from build123d import *

# Parameters (mm, degrees)
SKETCH1_W                  = 92
SKETCH1_H                  = 62
BOSS_EXTRUDE1_DEPTH        = 1
F_2_2_2_2_DIAMETER_HOLE2_D = 2.2


with BuildPart() as part:
    # Sketch1 → Boss-Extrude1 (new body)
    with BuildSketch(Plane.XY):
        with Locations((46, -31)):
            Rectangle(SKETCH1_W, SKETCH1_H)
    extrude(amount=-BOSS_EXTRUDE1_DEPTH)

    # Ø2.2 (2.2) Diameter Hole2 (through all)
    with Locations(Plane(origin=(0, 0, -1), x_dir=(-1, 0, 0), z_dir=(0, 0, -1))):
        with Locations((-79, -2), (-57, -2), (-35, -2), (-13, -2), (-13, -60), (-35, -60), (-57, -60), (-79, -60)):
            Hole(F_2_2_2_2_DIAMETER_HOLE2_D / 2)


solid = part.part
Input: part model. Units: mm. Frame: model coordinates. Give positions to 0.01 mm unless a question says otherwise; leave off trailing zeros. Order: outer loops, then holes, each group sorted by start corner. A loop starts at its lowest first (then second) coordinate and runs counter-clockwise, first axis right, second up. Notation, with made-up numbers: (28, -23.5) - (83, -23.5) arc R12 ccw to (83, -16.5) - close; hole circle Ø5 at (40.5, 70.5). An arc over 180 degrees is marked (long way). Answer as a JSON object with one key per item and string values. Group by question number.
Q1. Cut plane B-B, the plane y = -60. Output: boundary loops of the cut face in (x, z), then the cut area to 3 significant figures.
Q2. Line query: probe 1 along Y at (x, z) = (79, -0.7); probe 2 along Y at (x, z) = (12.5, -0.05). Output: solid intervals per line, ascending.
Q3. Mould query, pull axis Y, two halves, no side actions, for faces 1 (the face through (35.59, -59.07, -0.49)), 2 (the face through (45, -31, 0)). Classes: pulls with the +Y half, pulls with the -Y half, needs draft (parallel to the pull), parting line crosses it, or undercut.
Q4. First-contact query: pin 1 Ø1.8 at (x, y) = (35, -2) entering from -Z. Flat tip, straight axial feed; report the tip coordinate or a pass-through.
Q5. Cut plane A-A, the plane x = 35. Output: boundary loops of the cut face in (y, z).
Results:
{
 "1": {"outline": "(0, -1) - (11.9, -1) - (11.9, 0) - (0, 0) - close; (14.1, -1) - (33.9, -1) - (33.9, 0) - (14.1, 0) - close; (36.1, -1) - (55.9, -1) - (55.9, 0) - (36.1, 0) - close; (58.1, -1) - (77.9, -1) - (77.9, 0) - (58.1, 0) - close; (80.1, -1) - (92, -1) - (92, 0) - (80.1, 0) - close", "area": "83.2 mm^2"},
 "2": {"probe 1": "-62 to -61.1, -58.9 to -3.1, -0.9 to 0", "probe 2": "-62 to -60.98, -59.02 to -2.98, -1.02 to 0"},
 "3": {"face 1": "undercut", "face 2": "needs draft"},
 "4": {"pin 1": "through"},
 "5": {"outline": "(-62, -1) - (-61.1, -1) - (-61.1, 0) - (-62, 0) - close; (-58.9, -1) - (-3.1, -1) - (-3.1, 0) - (-58.9, 0) - close; (-0.9, -1) - (0, -1) - (0, 0) - (-0.9, 0) - close"}
}
